The listing builds one solid part. Answer for the finished solid, in the listing's coordinates (mm). Coordinates: 2 decimals unless noted, no trailing zeros. Write each loop counter-clockwise with the first axis right and the second up, starting at its lowest first coordinate (ties: lowest second). Pieces come first, ordered by that corner, then holes.
(1) The part is cut by section B-B on y = 0. Determine the outline of the cut face in (x, z).
(2) The part is cut by section C-C on z = 1.65. Give the number of separate pieces and of enclosed holes in the cut face, plus the area to 3 significant figures.
(3) Given P1, Ø1, axis at x = -9, z = 0.5, coming from the +Y side; P2, Ø6, axis at x = -41.5, y = 12, coming from the -Z side; P3, Ø4.5, axis at x = -14.14, y = 14.14, coming from the +Z side; P4, Ø0.9, axis at y = -2, z = 2, coming from the +X side, each flat-ended and moving along its own axis, determine where each tip first touches the part or whether it passes through.
(4) Straight lines are drawn through the part: line 1 (Y direction, x = 0, z = 1.45); line 2 (Y direction, x = -14.5, z = 0.9); line 3 (X direction, y = 13, z = 0.1). For each, find the intervals that lie inside material, in ascending order.
(5) The part is cut by section A-A on x = 0. Determine the outline of the cut face in (y, z).
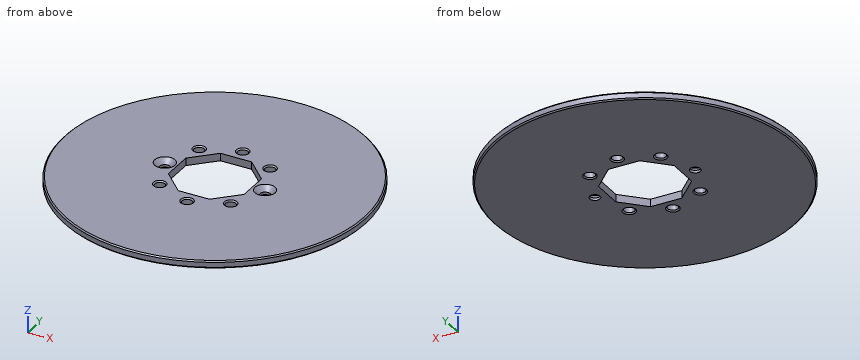
Autodesk Inventor part; units mm, degrees
ref_plane "YZ Plane" through (0, 0, 0) normal (1, 0, 0) x (0, 1, 0)
ref_plane "XZ Plane" through (0, 0, 0) normal (0, 1, 0) x (-1, 0, 0)
ref_plane "XY Plane" through (0, 0, 0) normal (0, 0, 1) x (1, 0, 0)
sketch "Sketch1" plane through (0, 0, 0) normal (0, 0, 1) x (1, 0, 0)
  circle A0 centre (0, 0) radius 60
  dimension "d0" = 120
extrude "Extrusion1" add sketch "Sketch1" along normal blind 3
sketch "Sketch3" plane through (0, 0, 3) normal (0, 0, 1) x (1, 0, 0)
  line L0 (-15.1, 6.2546) -> (-6.2546, 15.1)
  line L1 (-15.1, -6.2546) -> (-15.1, 6.2546)
  line L2 (-6.2546, -15.1) -> (-15.1, -6.2546)
  line L3 (6.2546, -15.1) -> (-6.2546, -15.1)
  line L4 (15.1, -6.2546) -> (6.2546, -15.1)
  line L5 (15.1, 6.2546) -> (15.1, -6.2546)
  line L6 (6.2546, 15.1) -> (15.1, 6.2546)
  line L7 (-6.2546, 15.1) -> (6.2546, 15.1)
  point P0 (0, 0)
  point P1 (0, 0)
extrude "Extrusion3" cut sketch "Sketch3" against normal through all
sketch "Sketch4" plane through (0, 0, 3) normal (0, 0, 1) x (1, 0, 0)
  line L0 (0, 0) -> (41.4197, 0)
  circle A0 centre (20, 0) radius 2.05
  circle A1 centre (20, 0) radius 2.05
  circle A2 centre (14.1421, 14.1421) radius 2.05
  circle A3 centre (0, 20) radius 2.05
  circle A4 centre (-14.1421, 14.1421) radius 2.05
  circle A5 centre (-20, 0) radius 2.05
  circle A6 centre (-14.1421, -14.1421) radius 2.05
  circle A7 centre (0, -20) radius 2.05
  circle A8 centre (14.1421, -14.1421) radius 2.05
  dimension "d26" = 360
  dimension "d27" = 4.1
extrude "Extrusion4" cut sketch "Sketch4" against normal through all
chamfer "Chamfer1" distance 2 angle 45 2 edges at (-22.05, 0, 3) (17.95, 0, 3)
chamfer "Chamfer2" distance 0.5 angle 45 14 edges at (-60, 0, 3) (-60, 0, 0) (-2.05, -20, 3) (12.0921, -14.1421, 3) (-16.1921, -14.1421, 3) (-16.1921, 14.1421, 3) (-2.05, 20, 3) (12.0921, 14.1421, 3) (-16.1921, -14.1421, 0) (-2.05, -20, 0) (12.0921, -14.1421, 0) (-16.1921, 14.1421, 0) (-2.05, 20, 0) (12.0921, 14.1421, 0)
properties part number "spool_side"
Model answer:
1. outline: (-60, 0.5) - (-59.5, 0) - (-22.05, 0) - (-22.05, 1) - (-24.05, 3) - (-59.5, 3) - (-60, 2.5) - close; (-17.95, 0) - (-15.1, 0) - (-15.1, 3) - (-15.95, 3) - (-17.95, 1) - close; (15.1, 0) - (17.95, 0) - (17.95, 1) - (15.95, 3) - (15.1, 3) - close; (22.05, 0) - (59.5, 0) - (60, 0.5) - (60, 2.5) - (59.5, 3) - (24.05, 3) - (22.05, 1) - close
2. separate pieces: 1
2. enclosed holes: 9
2. area: 10,400 mm2
3. P1: stops at y = 59.39
3. P2: stops at z = 0
3. P3: stops at z = 2.7
3. P4: stops at x = 59.98
4. line 1: y = -60 to -22.05, -17.95 to -15.1, 15.1 to 17.95, 22.05 to 60
4. line 2: y = -58.22 to -16.16, -12.12 to -6.85, 6.85 to 12.12, 16.16 to 58.22
4. line 3: x = -58.16 to -16.31, -11.97 to -8.35, 8.35 to 11.97, 16.31 to 58.16
5. outline: (-60, 0.5) - (-59.5, 0) - (-22.55, 0) - (-22.05, 0.5) - (-22.05, 2.5) - (-22.55, 3) - (-59.5, 3) - (-60, 2.5) - close; (-17.95, 0.5) - (-17.45, 0) - (-15.1, 0) - (-15.1, 3) - (-17.45, 3) - (-17.95, 2.5) - close; (15.1, 0) - (17.45, 0) - (17.95, 0.5) - (17.95, 2.5) - (17.45, 3) - (15.1, 3) - close; (22.05, 0.5) - (22.55, 0) - (59.5, 0) - (60, 0.5) - (60, 2.5) - (59.5, 3) - (22.55, 3) - (22.05, 2.5) - close
